Source: CAD feature listing. Evaluate the final solid. Frame: model axes, mm. Give positions to 0.01 mm unless a question says otherwise; leave off trailing zeros. Order: outer loops, then holes, each group sorted by start corner. A loop starts at its lowest first (then second) coordinate and runs counter-clockwise, first axis right, second up. Notation, with made-up numbers: (34.5, -39) -> (52.5, -39) arc R23 ccw to (52.5, -10) -> close; hole circle Ø9 at (66, -5). An arc over 180 degrees is marked (long way). Use one line per item in the form item = value. Start each with the question number.
Autodesk Inventor part; units mm, degrees
ref_plane "YZ Plane" through (0, 0, 0) normal (1, 0, 0) x (0, 1, 0)
ref_plane "XZ Plane" through (0, 0, 0) normal (0, 1, 0) x (-1, 0, 0)
ref_plane "XY Plane" through (0, 0, 0) normal (0, 0, 1) x (1, 0, 0)
sketch "main" plane through (0, 0, 0) normal (0, 0, 1) x (1, 0, 0)
  line L0 (10.9249, 53.4086) -> (-34.6395, -10.8755)
  line L1 (28.7127, 49.7366) -> (28.7127, -13.7634)
  arc A0 (16.1055, 56.0866) -> (10.9249, 53.4086) centre (16.1055, 49.7366) ccw
  line L2 (22.3627, 56.0866) -> (16.1055, 56.0866)
  arc A1 (28.7127, 49.7366) -> (22.3627, 56.0866) centre (22.3627, 49.7366) ccw
  arc A2 (26.9969, -18.1047) -> (28.7127, -13.7634) centre (22.3627, -13.7634) ccw
  arc A3 (-34.6395, -10.8755) -> (-34.7267, -14.4179) centre (-32.0492, -12.7116) ccw
  line L3 (-2.7465, -49.8547) -> (26.9969, -18.1047)
  circle A4 centre (-7.3807, -45.5134) radius 2.0955
  arc A5 (-12.7358, -48.926) -> (-2.7465, -49.8547) centre (-7.3807, -45.5134) ccw
  line L4 (-34.7267, -14.4179) -> (-12.7358, -48.926)
  circle A6 centre (-7.3807, -20.1134) radius 2.0955
  circle A7 centre (22.3627, 49.7366) radius 2.1844
  circle A8 centre (22.3627, -13.7634) radius 2.1844
  circle A9 centre (-7.3807, -32.8134) radius 2.0955
  point P0 (3.7494, 2.3687)
  point P1 (14.8443, 56.0866)
  dimension "d0" = 6.35
  dimension "d1" = 4.191
  dimension "d2" = 12.7
  dimension "d3" = 3.175
  dimension "d4" = 4.3688
  dimension "d5" = 4.3688
  dimension "d6" = 4.191
  dimension "d7" = 4.191
sketch "Sketch1" plane through (0, 0, 0) normal (0, 0, 1) x (1, 0, 0)
  line L0 (-73.522, 18.3056) -> (-9.2379, -27.2588)
  line L1 (-69.85, 36.0934) -> (-6.35, 36.0934)
  arc A0 (-76.2, 23.4862) -> (-73.522, 18.3056) centre (-69.85, 23.4862) ccw
  line L2 (-76.2, 29.7434) -> (-76.2, 23.4862)
  arc A1 (-69.85, 36.0934) -> (-76.2, 29.7434) centre (-69.85, 29.7434) ccw
  arc A2 (-2.0087, 34.3776) -> (-6.35, 36.0934) centre (-6.35, 29.7434) ccw
  arc A3 (-9.2379, -27.2588) -> (-5.6956, -27.346) centre (-7.4019, -24.6685) ccw
  line L3 (29.7413, 4.6342) -> (-2.0087, 34.3776)
  circle A4 centre (25.4, 0) radius 2.0955
  arc A5 (28.8126, -5.3551) -> (29.7413, 4.6342) centre (25.4, 0) ccw
  line L4 (-5.6956, -27.346) -> (28.8126, -5.3551)
  circle A6 centre (0, 0) radius 2.0955
  circle A7 centre (-69.85, 29.7434) radius 2.1844
  circle A8 centre (-6.35, 29.7434) radius 2.1844
  circle A9 centre (12.7, 0) radius 2.0955
extrude "Extrusion1" add sketch "Sketch1" along normal blind 1.5875
properties part number "sled" material "Acetal Resin, White"
1) Cut plane C-C, the plane y = 0. Return the cut outline in (x, z), plus the area to 3 significant figures.
2) Cut plane B-B, the plane x = 25.4. Return the cut outline in (y, z).
3) Pin query (flat end, axial travel): pin 1 (5 mm diameter, centred on x = -6.35, y = 29.74, fed in from -Z); pin 2 (8 mm diameter, centred on x = -54.5, y = -4, fed in from -Z). Return the tip coordinate at first contact, or that it passes through.
4) Cut plane A-A, the plane z = 0.4. Return the cut outline in (x, y).
5) Draft query along Y for faces 1 (the face through (-23, 12, 0)), 2 (the face through (14.636, 0.803, 0.783)), 3 (the face through (-41.83, -4.16, 0.78)). Return one class per face: +Y half, -Y half, draft (parallel to the pull), parting line (faces both ways), or undercut.
6) Cut plane D-D, the plane x = 12.7. Return the cut outline in (y, z).
7) Material intervals for probe 1 along X at (y, z) = (29, 1.1); probe 2 along Y at (x, z) = (25.4, 1.05); probe 3 along Y at (x, z) = (0, 0.4), sorted ascending.
Output values:
q1.outline = (-47.7, 0) -> (-2.1, 0) -> (-2.1, 1.59) -> (-47.7, 1.59) -> close; (2.1, 0) -> (10.6, 0) -> (10.6, 1.59) -> (2.1, 1.59) -> close; (14.8, 0) -> (23.3, 0) -> (23.3, 1.59) -> (14.8, 1.59) -> close; (27.5, 0) -> (31.75, 0) -> (31.75, 1.59) -> (27.5, 1.59) -> close
q1.area = 106 mm^2
q2.outline = (-7.53, 0) -> (-2.1, 0) -> (-2.1, 1.59) -> (-7.53, 1.59) -> close; (2.1, 0) -> (8.7, 0) -> (8.7, 1.59) -> (2.1, 1.59) -> close
q3.pin_1 = 0
q3.pin_2 = through
q4.outline = (-76.2, 23.49) arc R6.35 ccw to (-73.52, 18.31) -> (-9.24, -27.26) arc R3.17 ccw to (-5.7, -27.35) -> (28.81, -5.36) arc R6.35 ccw to (29.74, 4.63) -> (-2.01, 34.38) arc R6.35 ccw to (-6.35, 36.09) -> (-69.85, 36.09) arc R6.35 ccw to (-76.2, 29.74) -> close; hole circle Ø4.37 at (-69.85, 29.74); hole circle Ø4.37 at (-6.35, 29.74); hole circle Ø4.19 at (0, 0); hole circle Ø4.19 at (12.7, 0); hole circle Ø4.19 at (25.4, 0)
q5.face_1 = draft
q5.face_2 = undercut
q5.face_3 = -Y half
q6.outline = (-15.62, 0) -> (-2.1, 0) -> (-2.1, 1.59) -> (-15.62, 1.59) -> close; (2.1, 0) -> (20.6, 0) -> (20.6, 1.59) -> (2.1, 1.59) -> close
q7.probe_1 = -76.2 to -71.9, -67.8 to -8.4, -4.3 to 3.73
q7.probe_2 = -7.53 to -2.1, 2.1 to 8.7
q7.probe_3 = -23.72 to -2.1, 2.1 to 32.5
